Verification items for the finished model (mm, model axes). A direction names the side the tool comes from. Give positions to 0.01 mm unless a question says otherwise; leave off trailing zeros. Loops run counter-clockwise (first coordinate to the right, second up) from the corner with the lowest first, then second, coordinate; pieces in that order, holes last. Notation, with made-up numbers: (10, -37.75) - (27, -37.75) arc R28 ccw to (27, -17.75) - close; hole circle Ø6 at (56, 49). An arc over 180 degrees is marked (long way). Answer in a Markdown table with one row per item.
```python
from build123d import *

# Parameters (mm, degrees)
F0_W     = 110.554024
F0_H     = 110.554024
F1_DEPTH = 25
F2_R     = 11.5
F3_DEPTH = 25
F4_R     = 4.674091
F5_DEPTH = 25


with BuildPart() as f1:
    # F0 (on Front) → F1 (new body, symmetric)
    with BuildSketch(Plane.XZ):
        Rectangle(F0_W, F0_H)
    extrude(amount=F1_DEPTH, both=True)

    # F2 (on Front) → F3 (cut, through all)
    with BuildSketch(Plane.XZ):
        Circle(F2_R)
    extrude(amount=F3_DEPTH, mode=Mode.SUBTRACT)

    # F4 (on face) → F5 (cut, through all)
    with BuildSketch(Plane.XZ):
        Circle(F4_R)
    extrude(amount=-F5_DEPTH, mode=Mode.SUBTRACT)


solid = f1.part
```
Q1. Tool access check on faces 4 (the face through (55.277, 0, -1)), 5 (the face through (-1.5, -12.3, 11.4)). Record the directions out of +Z, -Z, +X, -X, +Y, -Y that give a thin tool (end or side, any length) a straight path to the whole face; none if there is none.
Completed:
| item | result |
|---|---|
| face 4 | +Z, -Z, +X, +Y, -Y |
| face 5 | -Y |
Q2. Go/stop test with a flat-tipped pin: P1, Ø18.5, axis at x = -4, z = 4.5, coming from the -Y side. Record where the tip stops, or that it passes through.
Completed:
| item | result |
|---|---|
| P1 | y = -25 |
Q3. Draft check along Z on faces 1 (the face through (-13, -25, 1)), 2 (the face through (5, 0, 0)), 3 (the face through (-1, 0, -55.277)). Enter one of: +Z half, -Z half, draft (parallel to the pull), parting line (faces both ways), or undercut.
Completed:
| item | result |
|---|---|
| face 1 | draft |
| face 2 | undercut |
| face 3 | -Z half |
Q4. Sectioned sample at A-A (z = 0). Record the cut outline in (x, y), and give its area (3 significant figures).
Completed:
| item | result |
|---|---|
| outline | (-55.28, -25) - (-11.5, -25) - (-11.5, 0) - (-4.67, 0) - (-4.67, 25) - (-55.28, 25) - close; (4.67, 0) - (11.5, 0) - (11.5, -25) - (55.28, -25) - (55.28, 25) - (4.67, 25) - close |
| area | 4,720 mm^2 |
Q5. Sectioned sample at B-B (x = 0). Record the cut outline in (y, z).
Completed:
| item | result |
|---|---|
| outline | (-25, -55.28) - (25, -55.28) - (25, -4.67) - (0, -4.67) - (0, -11.5) - (-25, -11.5) - close; (-25, 11.5) - (0, 11.5) - (0, 4.67) - (25, 4.67) - (25, 55.28) - (-25, 55.28) - close |
Q6. Sectioned sample at C-C (y = -14.5). Record the cut outline in (x, z), and give its area (3 significant figures).
Completed:
| item | result |
|---|---|
| outline | (-55.28, -55.28) - (55.28, -55.28) - (55.28, 55.28) - (-55.28, 55.28) - close; hole circle Ø23 at (0, 0) |
| area | 11,800 mm^2 |
Q7. Thickness scan on line 1 (Z direction, x = 0, y = -7.5); line 2 (Z direction, x = 0, y = 7.5). Record the ranges inside material, lowest first.
Completed:
| item | result |
|---|---|
| line 1 | -55.28 to -11.5, 11.5 to 55.28 |
| line 2 | -55.28 to -4.67, 4.67 to 55.28 |
